Check sheet for the drawn part. Datum: minimum x, y, z corner. Units: mm. A direction names the side the tool comes from. Round coordinates to 2 decimals unless told otherwise and drop trailing zeros. Write each loop counter-clockwise with the first axis right and the second up, starting at its lowest first coordinate (ties: lowest second). Pieces come first, ordered by that corner, then holes. Notation, with made-up numbers: (-9.5, 64.5) - (24.5, 64.5) arc R17 ccw to (24.5, 84.5) - close; hole circle Ø2 at (40, -34.75). An arc over 180 degrees is marked (long way). Answer as a JSON object with one key per item and string values.
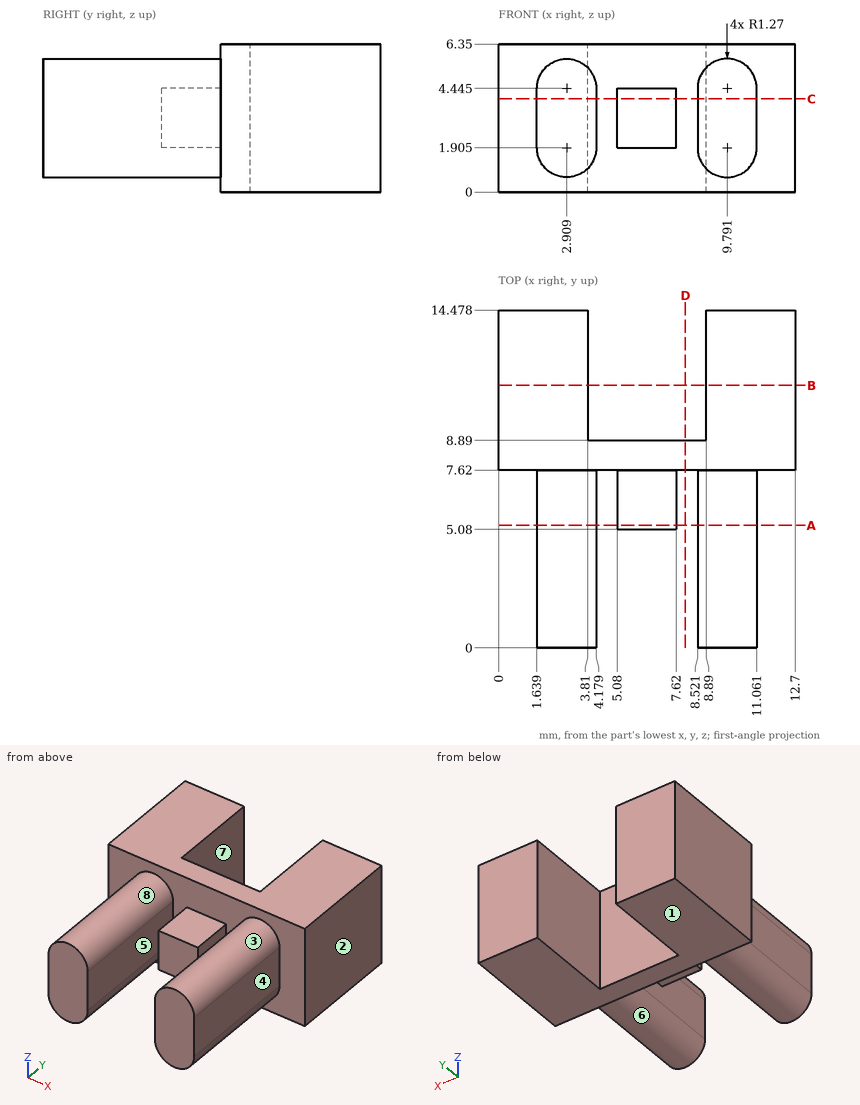
1. Cross-section at D-D (x = 8). Record the boundary of the cut face in (y, z).
Completed:
{"outline": "(7.62, 0) - (8.89, 0) - (8.89, 6.35) - (7.62, 6.35) - close"}
2. Cross-section at C-C (z = 4). Record the boundary of the cut face in (x, y).
Completed:
{"outline": "(0, 7.62) - (1.64, 7.62) - (1.64, 0) - (4.18, 0) - (4.18, 7.62) - (5.08, 7.62) - (5.08, 5.08) - (7.62, 5.08) - (7.62, 7.62) - (8.52, 7.62) - (8.52, 0) - (11.06, 0) - (11.06, 7.62) - (12.7, 7.62) - (12.7, 14.48) - (8.89, 14.48) - (8.89, 8.89) - (3.81, 8.89) - (3.81, 14.48) - (0, 14.48) - close"}
3. Material ranges on probe 1 along X at (y, z) = (6.75, 2.25); probe 2 along X at (y, z) = (12.75, 5.5); probe 3 along X at (y, z) = (3.25, 3.75), recorded low to high. Write a range as from..to.
Completed:
{"probe 1": "x = 1.64..4.18, 5.08..7.62, 8.52..11.06", "probe 2": "x = 0..3.81, 8.89..12.7", "probe 3": "x = 1.64..4.18, 8.52..11.06"}
4. Cross-section at B-B (y = 11.25). Record the boundary of the cut face in (x, z).
Completed:
{"outline": "(0, 0) - (3.81, 0) - (3.81, 6.35) - (0, 6.35) - close; (8.89, 0) - (12.7, 0) - (12.7, 6.35) - (8.89, 6.35) - close"}
5. Access from +Z, -Z, +X, -X, +Y, -Y to the whole of each face (thin tool, end or side, straight path). Record for the marked faces 4, 5, 6, 7 and 8.
Completed:
{"face 4": "+Z, -Z, +X, -Y", "face 5": "+Z, -Z, -Y", "face 6": "-Z, -Y", "face 7": "+Z, -Z, +Y", "face 8": "+Z, -Y"}
6. Cross-section at A-A (y = 5.25). Record the boundary of the cut face in (x, z) (3 decimals), plus the area to 3 significant figures.
Completed:
{"outline": "(1.639, 1.905) arc R1.27 ccw to (4.179, 1.905) - (4.179, 4.445) arc R1.27 ccw to (1.639, 4.445) - close; (5.08, 1.905) - (7.62, 1.905) - (7.62, 4.445) - (5.08, 4.445) - close; (8.521, 1.905) arc R1.27 ccw to (11.061, 1.905) - (11.061, 4.445) arc R1.27 ccw to (8.521, 4.445) - close", "area": "29.5 mm^2"}
7. Mould release check, pull along X, two halves, no side actions. Record for the marked faces 1, 2 and 3: released by +X, released by -X, zero draft, split by the parting line, or undercut.
Completed:
{"face 1": "zero draft", "face 2": "released by +X", "face 3": "undercut"}
8. Go/stop test with flat-tipped pins: pin 1 (1 mm diameter, centred on x = 2, y = 5.5, fed in from +Z); pin 2 (2 mm diameter, centred on y = 4, z = 3, fed in from +X); pin 3 (0.8 mm diameter, centred on y = 2.5, z = 3.5, fed in from -X). Record where each tip stops, or that it passes through.
Completed:
{"pin 1": "stops at z = 5.65", "pin 2": "stops at x = 11.06", "pin 3": "stops at x = 1.64"}
